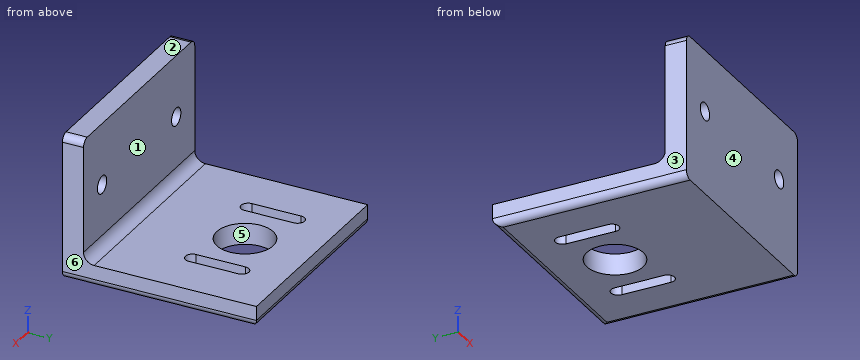
```python
from build123d import *

# Parameters (mm, degrees)
SKETCH2_W           = 60
SKETCH2_H           = 35
BOSS_EXTRUDE1_DEPTH = 6
SKETCH3_W           = 60
SKETCH3_H           = 55
BOSS_EXTRUDE2_DEPTH = 6
SKETCH4_R           = 8
CUT_EXTRUDE1_DEPTH  = 72.763500472
CUT_EXTRUDE2_DEPTH  = 72.763500472
SKETCH6_R           = 2.5
CUT_EXTRUDE3_DEPTH  = 6
FILLET1_R           = 2
FILLET2_R           = 3


with BuildPart() as part:
    # Sketch2 → Boss-Extrude1 (new body)
    with BuildSketch(Plane(origin=(0, 0, 0), x_dir=(1, 0, 0), z_dir=(0, 1, 0))):
        Rectangle(SKETCH2_W, SKETCH2_H)
    extrude(amount=BOSS_EXTRUDE1_DEPTH)

    # Sketch3 → Boss-Extrude2 (add)
    with BuildSketch(Plane(origin=(0, 0, -17.5), x_dir=(-1, 0, 0), z_dir=(0, 0, -1))):
        with Locations((0, 27.5)):
            Rectangle(SKETCH3_W, SKETCH3_H)
    extrude(amount=BOSS_EXTRUDE2_DEPTH)

    # Sketch4 → Cut-Extrude1 (cut, through all)
    with BuildSketch(Plane.XY.offset(-17.5)):
        with Locations((0, 36)):
            Circle(SKETCH4_R)
    extrude(amount=-CUT_EXTRUDE1_DEPTH, mode=Mode.SUBTRACT)

    # Sketch5 → Cut-Extrude2 (cut, through all)
    with BuildSketch(Plane.XY.offset(-17.5)):
        with BuildLine():
            Line((-13, 43), (-13, 29))
            ThreePointArc((-13, 29), (-15, 27), (-17, 29))
            Line((-17, 29), (-17, 43))
            ThreePointArc((-17, 43), (-15, 45), (-13, 43))
        make_face()
        with BuildLine():
            Line((17, 43), (17, 29))
            ThreePointArc((17, 29), (15, 27), (13, 29))
            Line((13, 29), (13, 43))
            ThreePointArc((13, 43), (15, 45), (17, 43))
        make_face()
    extrude(amount=-CUT_EXTRUDE2_DEPTH, mode=Mode.SUBTRACT)

    # Sketch6 → Cut-Extrude3 (cut)
    with BuildSketch(Plane(origin=(0, 6, 0), x_dir=(1, 0, 0), z_dir=(0, 1, 0))):
        with Locations(Location((-20, 0, 0), (0, 0, 270))):
            Circle(SKETCH6_R)
        with Locations(Location((20, 0, 0), (0, 0, 270))):
            Circle(SKETCH6_R)
    extrude(amount=-CUT_EXTRUDE3_DEPTH, mode=Mode.SUBTRACT)

    # Fillet1
    fillet1_edges = [part.edges().sort_by_distance(p)[0] for p in [
        (30, 27.5, -23.5),
        (-30, 27.5, -23.5),
        (0, 55, -23.5),
        (30, 3, 17.5),
        (-30, 3, 17.5),
    ]]
    fillet(fillet1_edges, radius=FILLET1_R)

    # Fillet2
    fillet2_edges = [part.edges().sort_by_distance(p)[0] for p in [
        (0, 6, -17.5),
    ]]
    fillet(fillet2_edges, radius=FILLET2_R)


solid = part.part
```
Design review of the part built by this model. Coordinates are the model's own, in mm. Face numbers are marked on the shaded views. A direction names the side the tool comes from. Give positions to 0.01 mm unless a question says otherwise; leave off trailing zeros. Loops run counter-clockwise (first coordinate to the right, second up) from the corner with the lowest first, then second, coordinate; pieces in that order, holes last. Notation, with made-up numbers: M -8,-34.5 L 18,-34.5 A11 cw 18,-24.5 Z; hole C 60,72 d4. An arc over 180 degrees is marked long. Return JSON: item names as keys, results as strings. Group by question number.
Item 1: We need section B-B (x = 20). Give the boundary of the cut face in (y, z), and give its area (3 significant figures).
Item 2: Tool access review of the marked faces 1 and 2: name each direction out of +Z, -Z, +X, -X, +Y, -Y from which nothing blocks a thin tool from reaching the whole face with its end or side.
Item 3: Insertion check: pin 1 Ø8 at (x, z) = (20.5, -10) entering from +Y; pin 2 Ø1.5 at (x, y) = (-0.5, 47) entering from +Z; pin 3 Ø9.5 at (x, y) = (0, 36) entering from -Z. Each pin has a flat end and moves straight along its axis. Give the tip position at first contact, or say it passes through.
Item 4: We need section D-D (x = -10). Give the boundary of the cut face in (y, z).
Item 5: We need section C-C (z = 1). Give the boundary of the cut face in (x, y).
Item 6: Mouldability with a two-part tool opening along X and no side actions: class the marked faces 3, 4, 5 and 6 as released by +X, released by -X, zero draft, split by the parting line, or undercut.
Item 7: We need section A-A (y = 36). Give the boundary of the cut face in (x, z), and give its area (3 significant figures).
Item 8: For probe 1 along X at (y, z) = (3, 0); probe 2 along Y at (x, z) = (0, -20.2); probe 3 along Y at (x, z) = (24.5, -6), list the stretches that pass through material, from the lowest coordinate up.
Output:
{
 "1": {"outline": "M 0,-23.5 L 53,-23.5 A2 ccw 55,-21.5 L 55,-17.5 L 9,-17.5 A3 cw 6,-14.5 L 6,-2.5 L 0,-2.5 Z; M 0,2.5 L 6,2.5 L 6,17.5 L 0,17.5 Z", "area": "511 mm^2"},
 "2": {"face 1": "+Z, +X, -X, +Y", "face 2": "+Z, +X, -X, +Y, -Y"},
 "3": {"pin 1": "stops at y = 6", "pin 2": "stops at z = -17.5", "pin 3": "passes through"},
 "4": {"outline": "M 0,-23.5 L 53,-23.5 A2 ccw 55,-21.5 L 55,-17.5 L 9,-17.5 A3 cw 6,-14.5 L 6,17.5 L 0,17.5 Z"},
 "5": {"outline": "M -30,0 L -22.29,0 L -22.29,6 L -30,6 Z; M -17.71,0 L 17.71,0 L 17.71,6 L -17.71,6 Z; M 22.29,0 L 30,0 L 30,6 L 22.29,6 Z"},
 "6": {"face 3": "released by -X", "face 4": "zero draft", "face 5": "undercut", "face 6": "released by +X"},
 "7": {"outline": "M -30,-21.5 A2 ccw -28,-23.5 L -17,-23.5 L -17,-17.5 L -30,-17.5 Z; M -13,-23.5 L -8,-23.5 L -8,-17.5 L -13,-17.5 Z; M 8,-23.5 L 13,-23.5 L 13,-17.5 L 8,-17.5 Z; M 17,-23.5 L 28,-23.5 A2 ccw 30,-21.5 L 30,-17.5 L 17,-17.5 Z", "area": "214 mm^2"},
 "8": {"probe 1": "x = -30 to -22.5, -17.5 to 17.5, 22.5 to 30", "probe 2": "y = 0 to 28, 44 to 55", "probe 3": "y = 0 to 6"}
}
